Design review of the part built by this model. Coordinates are the model's own, in mm. A direction names the side the tool comes from. Coordinates: 2 decimals unless noted, no trailing zeros. Loops run counter-clockwise (first coordinate to the right, second up) from the corner with the lowest first, then second, coordinate; pieces in that order, holes last.
Q1. Wall thickness on probe 1 along X at (y, z) = (10.25, 22.5); probe 2 along Z at (x, y) = (24.75, 6.75); probe 3 along Y at (x, z) = (22.75, 18.5): over which ranges is each line inside the solid? List them lowest first.
Q2. Add section A-A on x = 10. Give the boundary of the cut face in (y, z).
Q3. Machinability: for faces 1 (the face through (12, 0, 15)), 2 (the face through (-1, 6, 8.75)), 3 (the face through (9, -1, 7)), 4 (the face through (22.048, 0.713, 4.436)), which of the approach directions +Z, -Z, +X, -X, +Y, -Y give a long, thin tool a straight path to every point of the face, cutting with its end or side? Answer none if there is none.
Q4. Add section C-C on z = 7.75. Give the boundary of the cut face in (x, y).
Q5. Add section B-B on y = -0.5. Give the boundary of the cut face in (x, z), and give its area (3 significant figures).
Q6. For P1, Ø1, axis at x = 21.5, z = 26, coming from the +Y side; P2, Ø2.5, axis at y = 4.78, z = 24.97, coming from the +X side; P3, Ø5, axis at x = 10, z = 4.5, coming from the +Y side, all flat-tipped, find the tip position at first contact; note any pin that passes through.
Q7. Draft analysis for pull direction Z (two halves, no side actions). For faces 5 (the face through (-1, 12, 4)), 6 (the face through (-1, 6, 21.25)), 7 (the face through (11.2, -0.4, 0)), state which applies: released by +Z, released by -Z, zero draft, split by the parting line, or undercut.
Q8. Add section D-D on y = 10. Give the boundary of the cut face in (x, z).
```python
from build123d import *

# Parameters (mm, degrees)
EXTRUDE_1_DEPTH     = 30
SKETCH_2_W          = 12.5
SKETCH_2_H          = 12
CUT_EXTRUDE_1_DEPTH = 28.8
CUT_EXTRUDE_2_REACH = 5
MM_PRESS_1_D        = 3
FILLET_1_R          = 2.5


with BuildPart() as part:
    # 草图1 → 凸台-拉伸1 (new body)
    with BuildSketch(Plane.XY):
        Polygon((0, 0), (0, 12), (-3, 12), (-3, -3), (25.8, -3), (25.8, 12), (22.8, 12), (22.8, 0), align=None)
    extrude(amount=EXTRUDE_1_DEPTH)

    # 草图2 → 切除-拉伸1 (cut)
    with BuildSketch(Plane(origin=(25.8, 0, 0), x_dir=(0, 0, -1), z_dir=(1, 0, 0))):
        with Locations((-15, 6)):
            Rectangle(SKETCH_2_W, SKETCH_2_H)
    extrude(amount=-CUT_EXTRUDE_1_DEPTH, mode=Mode.SUBTRACT)

    # 草图3 → 切除-拉伸2 (cut, up to next)
    with BuildSketch(Plane(origin=(0, 0, 0), x_dir=(1, 0, 0), z_dir=(0, 1, 0)), mode=Mode.PRIVATE) as cut_extrude_2_sk1:
        with BuildLine():
            Line((11, -4.647050091), (11, -8.647050091))
            ThreePointArc((11, -8.647050091), (10, -9.647050091), (9, -8.647050091))
            Line((9, -8.647050091), (9, -4.647050091))
            ThreePointArc((9, -4.647050091), (10, -3.647050091), (11, -4.647050091))
        make_face()
    cut_extrude_2_tool1 = extrude(cut_extrude_2_sk1.sketch, amount=-CUT_EXTRUDE_2_REACH, mode=Mode.PRIVATE) & part.part
    add(cut_extrude_2_tool1.solids().sort_by_distance((10, 0, 6.64705))[0], mode=Mode.SUBTRACT)
    # 草图3 → 切除-拉伸2 (cut, up to next)
    with BuildSketch(Plane(origin=(0, 0, 0), x_dir=(1, 0, 0), z_dir=(0, 1, 0)), mode=Mode.PRIVATE) as cut_extrude_2_sk2:
        with BuildLine():
            Line((11, -25.352949909), (11, -21.352949909))
            ThreePointArc((11, -21.352949909), (10, -20.352949909), (9, -21.352949909))
            Line((9, -21.352949909), (9, -25.352949909))
            ThreePointArc((9, -25.352949909), (10, -26.352949909), (11, -25.352949909))
        make_face()
    cut_extrude_2_tool2 = extrude(cut_extrude_2_sk2.sketch, amount=-CUT_EXTRUDE_2_REACH, mode=Mode.PRIVATE) & part.part
    add(cut_extrude_2_tool2.solids().sort_by_distance((10, 0, 23.35295))[0], mode=Mode.SUBTRACT)

    # 大小mm Press 暗销孔1 (through all)
    with Locations(Plane(origin=(-3, 140.185527162, 21.233815274), x_dir=(0, -0.020968354, -0.99978014), z_dir=(-1, 0, 0))):
        with Locations((20.608818994, 135.452556109), (-0.900285243, 135.452556109)):
            Hole(MM_PRESS_1_D / 2)

    # 圆角1
    fillet_1_edges = [part.edges().sort_by_distance(p)[0] for p in [
        (22.8, 0, 25.625),
        (0, 0, 25.625),
        (22.8, 0, 4.375),
        (0, 0, 4.375),
    ]]
    fillet(fillet_1_edges, radius=FILLET_1_R)


solid = part.part
```
Entries:
1. probe 1: x = -3 to 0, 22.8 to 25.8
1. probe 2: z = 0 to 8.75, 21.25 to 30
1. probe 3: y = -3 to 0
2. outline: (-3, 0) - (0, 0) - (0, 3.65) - (-3, 3.65) - close; (-3, 9.65) - (0, 9.65) - (0, 20.35) - (-3, 20.35) - close; (-3, 26.35) - (0, 26.35) - (0, 30) - (-3, 30) - close
3. face 1: +Y
3. face 2: +X, -X, +Y
3. face 3: +Y, -Y
3. face 4: +Z, -Z, +Y
4. outline: (-3, -3) - (9, -3) - (9, 0) - (2.5, 0) arc R2.5 cw to (0, 2.5) - (0, 12) - (-3, 12) - close; (11, -3) - (25.8, -3) - (25.8, 12) - (22.8, 12) - (22.8, 2.5) arc R2.5 cw to (20.3, 0) - (11, 0) - close
5. outline: (-3, 0) - (25.8, 0) - (25.8, 30) - (-3, 30) - close; hole (9, 4.65) arc R1 ccw to (11, 4.65) - (11, 8.65) arc R1 ccw to (9, 8.65) - close; hole (9, 21.35) arc R1 ccw to (11, 21.35) - (11, 25.35) arc R1 ccw to (9, 25.35) - close
5. area: 842 mm2
6. P1: stops at y = 0.67
6. P2: passes through
6. P3: stops at y = 0
7. face 5: zero draft
7. face 6: undercut
7. face 7: released by -Z
8. outline: (-3, 0) - (0, 0) - (0, 8.75) - (-3, 8.75) - close; (-3, 21.25) - (0, 21.25) - (0, 30) - (-3, 30) - close; (22.8, 0) - (25.8, 0) - (25.8, 8.75) - (22.8, 8.75) - close; (22.8, 21.25) - (25.8, 21.25) - (25.8, 30) - (22.8, 30) - close
